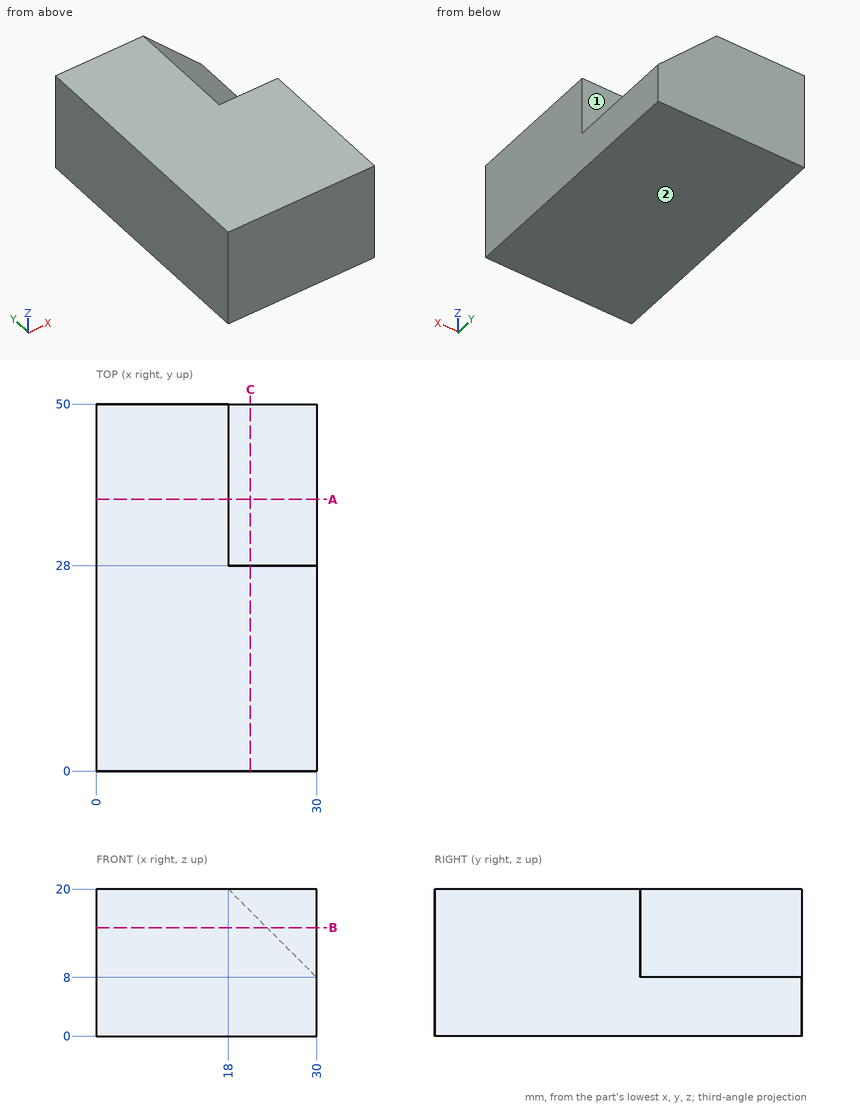
Verification items for this drawing (mm, ordinates from the low corner). A direction names the side the tool comes from. Coordinates: 2 decimals unless noted, no trailing zeros. Order: outer loops, then holes, each group sorted by start corner. A loop starts at its lowest first (then second) coordinate and runs counter-clockwise, first axis right, second up. Notation, with made-up numbers: (66.25, 45.25) - (111.25, 45.25) arc R13 cw to (111.25, 68.25) - close; hole circle Ø11 at (-20.75, -32). An arc over 180 degrees is marked (long way). Answer in a Markdown table with one row per item. Add a question column.
1. Section check C-C (x = 21). Enter the section's corners in (y, z), plus the area to 3 significant figures.
2. Section check B-B (z = 14.75). Enter the section's corners in (x, y).
3. Section check A-A (y = 37). Enter the section's corners in (x, z), plus the area to 3 significant figures.
4. Material ranges on L1, parallel to Y at x = 25.5, z = 19; L2, parallel to X at y = 32.5, z = 18; L3, parallel to X at y = 32.5, z = 14, recorded low to high. Write a range as [from, to].
5. Access from +Z, -Z, +X, -X, +Y, -Y to the whole of each face (thin tool, end or side, straight path). Record for the marked faces 1 and 2.
Data:
| question | item | result |
|---|---|---|
| 1 | outline | (0, 0) - (50, 0) - (50, 17) - (28, 17) - (28, 20) - (0, 20) - close |
| 1 | area | 934 mm² |
| 2 | outline | (0, 0) - (30, 0) - (30, 28) - (23.25, 28) - (23.25, 50) - (0, 50) - close |
| 3 | outline | (0, 0) - (30, 0) - (30, 8) - (18, 20) - (0, 20) - close |
| 3 | area | 528 mm² |
| 4 | L1 | y = [0, 28] |
| 4 | L2 | x = [0, 20] |
| 4 | L3 | x = [0, 24] |
| 5 | face 1 | +Z, +X, +Y |
| 5 | face 2 | -Z, +X, -X, +Y, -Y |
